```python
from build123d import *

# Parameters (mm, degrees)
F0_W     = 85
F0_H     = 56
F0_R     = 1.5
F1_DEPTH = 26
F2_W     = 69
F2_H     = 51
F3_DEPTH = 1
F4_W     = 3.6
F4_H     = 6
F5_DEPTH = 4


with BuildPart() as f1:
    # F0 (on Top) → F1 (new body)
    with BuildSketch(Plane.XY):
        with Locations((0, -3.51239704)):
            Rectangle(F0_W, F0_H)
        with Locations((-39, -28.01239704)):
            Circle(F0_R, mode=Mode.SUBTRACT)
        with Locations((39, -28.01239704)):
            Circle(F0_R, mode=Mode.SUBTRACT)
        with Locations((-39, 20.98760296)):
            Circle(F0_R, mode=Mode.SUBTRACT)
        with Locations((39, 20.98760296)):
            Circle(F0_R, mode=Mode.SUBTRACT)
    extrude(amount=F1_DEPTH)

    # F2 (on face) → F3 (join)
    with BuildSketch(Plane.XY.offset(26)):
        with Locations((-0.5440037453, -6.01239704)):
            Rectangle(F2_W, F2_H)
    extrude(amount=F3_DEPTH)

    # F4 (on face) → F5 (join)
    with BuildSketch(Plane.XY.offset(26)):
        with Locations((-39.2, 13.98760296)):
            Rectangle(F4_W, F4_H)
        with Locations((-39.2, 1.98760296)):
            Rectangle(F4_W, F4_H)
        with Locations((-39.2, -10.01239704)):
            Rectangle(F4_W, F4_H)
        with Locations((-39.2, -22.01239704)):
            Rectangle(F4_W, F4_H)
    extrude(amount=F5_DEPTH)


solid = f1.part
```
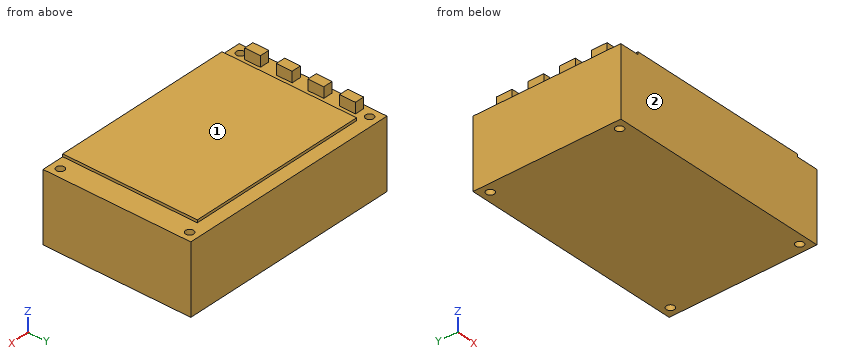
Input: part model. Units: mm. Frame: model coordinates. Face numbers are marked on the shaded views. A direction names the side the tool comes from. Round coordinates to 2 decimals unless told otherwise and drop trailing zeros. Write each loop counter-clockwise with the first axis right and the second up, starting at its lowest first coordinate (ties: lowest second). Pieces come first, ordered by that corner, then holes. Notation, with made-up numbers: (27.5, 53.5) -> (31.5, 53.5) arc R29 cw to (31.5, 74.5) -> close; hole circle Ø11 at (-38.75, 41). An arc over 180 degrees is marked (long way). Answer as CSV lines item,"result".
1. Reachability of the marked faces 1 and 2 from +Z, -Z, +X, -X, +Y, -Y: full face, straight path, thin tool, end or side. Return the list, or none.
Geometry says:
face 1,"+Z, +X, +Y, -Y"
face 2,"+Z, -Z, +X, -X, -Y"
2. Ray query, L1, parallel to Y at x = 39, z = 11.5; L2, parallel to Z at x = 13.5, y = 1.5. Return the intervals inside material, ascending. Write a range as [from, to].
Geometry says:
L1,"y = [-31.51, -29.51], [-26.51, 19.49], [22.49, 24.49]"
L2,"z = [0, 27]"
3. Section B-B (z = 28.25). Return the cut outline in (x, y).
Geometry says:
outline,"(-41, -25.01) -> (-37.4, -25.01) -> (-37.4, -19.01) -> (-41, -19.01) -> close; (-41, -13.01) -> (-37.4, -13.01) -> (-37.4, -7.01) -> (-41, -7.01) -> close; (-41, -1.01) -> (-37.4, -1.01) -> (-37.4, 4.99) -> (-41, 4.99) -> close; (-41, 10.99) -> (-37.4, 10.99) -> (-37.4, 16.99) -> (-41, 16.99) -> close"
4. Section D-D (x = -39). Return the cut outline in (y, z).
Geometry says:
outline,"(-31.51, 0) -> (-29.51, 0) -> (-29.51, 26) -> (-31.51, 26) -> close; (-26.51, 0) -> (19.49, 0) -> (19.49, 26) -> (16.99, 26) -> (16.99, 30) -> (10.99, 30) -> (10.99, 26) -> (4.99, 26) -> (4.99, 30) -> (-1.01, 30) -> (-1.01, 26) -> (-7.01, 26) -> (-7.01, 30) -> (-13.01, 30) -> (-13.01, 26) -> (-19.01, 26) -> (-19.01, 30) -> (-25.01, 30) -> (-25.01, 26) -> (-26.51, 26) -> close; (22.49, 0) -> (24.49, 0) -> (24.49, 26) -> (22.49, 26) -> close"
5. Contact query for flat-ended pins moving along their axis: P1, Ø0.8, axis at y = -16, z = 26.5, coming from the +X side; P2, Ø0.5, axis at x = 16, z = 26.5, coming from the +Y side; P3, Ø1.2, axis at y = 13, z = 28, coming from the +X side; P4, Ø2.5, axis at x = 39, y = 20.99, coming from the -Z side. Output: stop coordinate, or through.
Geometry says:
P1,"stops at x = 33.96"
P2,"stops at y = 19.49"
P3,"stops at x = -37.4"
P4,"passes through"
6. Section C-C (y = 3). Return the cut outline in (x, z).
Geometry says:
outline,"(-42.5, 0) -> (42.5, 0) -> (42.5, 26) -> (33.96, 26) -> (33.96, 27) -> (-35.04, 27) -> (-35.04, 26) -> (-37.4, 26) -> (-37.4, 30) -> (-41, 30) -> (-41, 26) -> (-42.5, 26) -> close"
7. Section A-A (x = 39). Return the cut outline in (y, z).
Geometry says:
outline,"(-31.51, 0) -> (-29.51, 0) -> (-29.51, 26) -> (-31.51, 26) -> close; (-26.51, 0) -> (19.49, 0) -> (19.49, 26) -> (-26.51, 26) -> close; (22.49, 0) -> (24.49, 0) -> (24.49, 26) -> (22.49, 26) -> close"
